from build123d import *

# Parameters (mm, degrees)
CIRPATTERN1_COUNT   = 3
CIRPATTERN1_ANGLE   = 180
SKETCH3_R           = 4.2
BOSS_EXTRUDE1_DEPTH = 0.25
CIRPATTERN2_COUNT   = 2
CIRPATTERN2_ANGLE   = 180


with BuildPart() as part:
    # Sketch1 → Revolve1 (revolve)
    with BuildSketch(Plane(origin=(0, 0, 0), x_dir=(0, 0, -1), z_dir=(1, 0, 0)), mode=Mode.PRIVATE) as revolve1_sk:
        with BuildLine():
            Line((16.603, 4.725), (17.238, 4.725))
            ThreePointArc((17.238, 4.725), (17.776815367, 4.501815367), (18, 3.963))
            Line((18, 3.963), (18, 3.381))
            Line((18, 3.381), (17.619, 3))
            Line((17.619, 3), (5.75, 3))
            Line((5.75, 3), (5.75, 2.238))
            Line((5.75, 2.238), (0, 2.238))
            Line((0, 2.238), (0, 4.2))
            Line((0, 4.2), (9, 4.2))
            Line((9, 4.2), (10.818653348, 5.25))
            Line((10.818653348, 5.25), (15.587, 5.25))
            Line((15.587, 5.25), (15.587, 4.2525))
            Line((15.587, 4.2525), (16.603, 4.2525))
            Line((16.603, 4.2525), (16.603, 4.725))
        make_face()
    revolve(revolve1_sk.sketch.rotate(Axis((0, 0, 0), (0, 0, -1)), 90), axis=Axis((0, 0, 0), (0, 0, -1)))


with BuildPart() as cirpattern1_1:
    # CirPattern1: pattern copy
    add(part.part.rotate(Axis((0, 0, 0), (1, 0, 0)), 1 * CIRPATTERN1_ANGLE / (CIRPATTERN1_COUNT - 1)))


with BuildPart() as cirpattern1_2:
    # CirPattern1: pattern copy
    add(part.part.rotate(Axis((0, 0, 0), (1, 0, 0)), 2 * CIRPATTERN1_ANGLE / (CIRPATTERN1_COUNT - 1)))


with BuildPart() as cirpattern1_1_1:
    # Body-Move/Copy1: moved
    add(cirpattern1_1.part.moved(Location((0, 0.25, 0))))

    # Sketch3 → Boss-Extrude1 (add)
    with BuildSketch(Plane(origin=(0, 0, 0), x_dir=(1, 0, 0), z_dir=(0, 1, 0))):
        Circle(SKETCH3_R)
    extrude(amount=BOSS_EXTRUDE1_DEPTH)


with BuildPart() as cut_revolve2_tool:
    # Sketch4 → Cut-Revolve2 (revolve)
    with BuildSketch(Plane(origin=(0, 0, 0), x_dir=(0, 0, -1), z_dir=(1, 0, 0))):
        Polygon((3, 17.869), (3.381, 18.25), (0, 18.25), (0, 0), (2.238, 0), (2.238, 6), (3, 6), align=None)
    revolve(axis=Axis((0, 0, 0), (0, 1, 0)))


with BuildPart() as part_1:
    add(part.part)

    # Cut-Revolve2: cut by cut_revolve2_tool
    add(cut_revolve2_tool.part, mode=Mode.SUBTRACT)


with BuildPart() as cirpattern1_1_2:
    add(cirpattern1_1_1.part)

    # Cut-Revolve2: cut by cut_revolve2_tool
    add(cut_revolve2_tool.part, mode=Mode.SUBTRACT)


with BuildPart() as cirpattern1_2_1:
    add(cirpattern1_2.part)

    # Cut-Revolve2: cut by cut_revolve2_tool
    add(cut_revolve2_tool.part, mode=Mode.SUBTRACT)


with BuildPart() as part_2:
    add(part_1.part)

    # Combine1: union CirPattern1_1, CirPattern1_2
    add(cirpattern1_1_2.part)
    add(cirpattern1_2_1.part)

    # Sketch5 → Cut-Revolve1 (revolve, cut)
    with BuildSketch(Plane(origin=(0, 0, 0), x_dir=(0, 0, -1), z_dir=(1, 0, 0)), mode=Mode.PRIVATE) as cut_revolve1_sk:
        Polygon((18, 3.381), (17.619, 3), (5.75, 3), (5.75, 2.238), (0, 2.238), (0, 0), (18, 0), align=None)
    cut_revolve1 = revolve(cut_revolve1_sk.sketch.rotate(Axis((0, 0, 0), (0, 0, -1)), 90), axis=Axis((0, 0, 0), (0, 0, -1)), mode=Mode.SUBTRACT)

    # CirPattern2: Cut-Revolve1 ×2 about axis
    cirpattern2_axis = Axis((-5.775, 0, 0), (1, 0, 0))
    for i in range(1, CIRPATTERN2_COUNT):
        add(cut_revolve1.rotate(cirpattern2_axis, i * CIRPATTERN2_ANGLE / (CIRPATTERN2_COUNT - 1)), mode=Mode.SUBTRACT)


solid = part_2.part
Build history of the part. All positions in model axes, mm. A direction names the side the tool comes from. Coordinates: 2 decimals unless noted, no trailing zeros. Write each loop counter-clockwise with the first axis right and the second up, starting at its lowest first coordinate (ties: lowest second). Pieces come first, ordered by that corner, then holes. Notation, with made-up numbers: (-33.5, -5) -> (-7.5, -5) arc R23 cw to (-7.5, 19) -> close; hole circle Ø4 at (5, 69). An arc over 180 degrees is marked (long way). Use CSV: the item, a comma, the result in double quotes. Start each with the question number.
Q1. Drill centre lines: probe 1 along X at (y, z) = (5.2, 0); probe 2 along Y at (x, z) = (0, -4); probe 3 along Z at (x, y) = (0.5, 4.5). Where is each one in solid material? Low to high.
Q2. Pull direction Y, two halves, no side cores. Call faces 1 (the flat face through (2, 4, -15.587)), 2 (the cylindrical face through (4.507, -1.419, -16.925)), 3 (the cylindrical face through (4.056, 16.352, -1.277)): released by +Y, released by -Y, zero draft, split by the parting line, or undercut.
Q3. Cut at A-A, the plane y = 7.25. List the corners of the cut face in (x, z), then the cut area to 3 significant figures.
Q4. Flat gauge pins, fed straight in: pin 1 Ø2.5 at (x, y) = (0, 0) entering from -Z; pin 2 Ø1 at (x, y) = (-4, 13.5) entering from +Z; pin 3 Ø3 at (x, y) = (1.5, -1) entering from -Z; pin 4 Ø3 at (y, z) = (1.5, -2) entering from +X. Where does each tip first touch, or does it go through?
Q5. 3-axis set-ups, long thin cutter, end or side, ignore diameter. For faces 4 (the flat face through (2, 15.837, 4)), 5 (the cylindrical face through (-0.65, -2.93, 11.6)), 6 (the flat face through (3, 18.25, -2)), 7 (the cylindrical face through (5, -1.6, -13.2)): which of +Z, -Z, +X, -X, +Y, -Y reach the whole face in a straight line?
Checked values:
1,probe 1,"x = -4.2 to -2.24, 2.24 to 4.2"
1,probe 2,"y = -4.2 to -2.24, 2.24 to 18.25"
1,probe 3,"z = -17.75 to -16.6, -15.59 to -9.57, -4.17 to -2.18, 2.18 to 4.17, 9.57 to 15.59, 16.6 to 17.75"
2,face 1,"zero draft"
2,face 2,"split by the parting line"
2,face 3,"undercut"
3,outline,"circle Ø8.4 at (0, 0); hole circle Ø6 at (0, 0)"
3,area,"27.1 mm²"
4,pin 1,"passes through"
4,pin 2,"stops at z = 3.91"
4,pin 3,"stops at z = -17.92"
4,pin 4,"stops at x = 4.2"
5,face 4,"none"
5,face 5,"+Z"
5,face 6,"+Z, -Z, +X, -X, +Y"
5,face 7,"-Z"
